Input: part model. Units: mm. Frame: model coordinates. A direction names the side the tool comes from. Coordinates: 2 decimals unless noted, no trailing zeros. Loops run counter-clockwise (first coordinate to the right, second up) from the corner with the lowest first, then second, coordinate; pieces in that order, holes last. Notation, with made-up numbers: M 84.25,43.5 L 123.25,43.5 A34 cw 123.25,73.5 Z; hole C 15.25,76.25 d5. An arc over 180 degrees is marked long. Use a Markdown table: item, result. Add a question column.
1. Pin query (flat end, axial travel): pin 1 (4 mm diameter, centred on x = 86.5, y = 23.5, fed in from +Z); pin 2 (4 mm diameter, centred on x = 32.5, y = 26.5, fed in from -Z); pin 3 (2 mm diameter, centred on x = 104, y = 16.5, fed in from +Z). Return the tip coordinate at first contact, or that it passes through.
2. Line query: L1, parallel to Y at x = 115, z = -24; L2, parallel to Z at x = 47.5, y = 40; L3, parallel to X at y = 10, z = 34.5. Output: solid intervals per line, ascending. Write a range as [from, to].
3. Section C-C on x = 112. Output: boundary loops of the cut face in (y, z), then the cut area to 3 significant figures.
4. Section A-A on y = 7. Output: boundary loops of the cut face in (x, z), then the cut area to 3 significant figures.
5. Set-up query: faces 1 (the flat face through (112, 22, 23)), 2 (the flat face through (105, 0, -23)). Return all of +Z, -Z, +X, -X, +Y, -Y with unobstructed straight access to the full face (end or side cutting, diameter ignored); none if empty.
6. Section D-D on y = 22. Output: boundary loops of the cut face in (x, z).
7. Section B-B on z = 46.5. Output: boundary loops of the cut face in (x, y).
```python
from build123d import *

# Parameters (mm, degrees)
SURFACESAB_DEPTH        = 150
SURFACESCD_DEPTH        = 80
SURFACESCD_DEPTH_BACK   = 70
CUT_EXTRUDE3_DEPTH      = 42.711375741
SURFACEE_DEPTH          = 130
CUT_EXTRUDE9_DEPTH      = 81
CUT_EXTRUDE9_DEPTH_BACK = 71
CUT_EXTRUDE10_DEPTH     = 150


with BuildPart() as part:
    # Sketch2 → SurfacesAB (new body)
    with BuildSketch(Plane(origin=(0, 0, 0), x_dir=(0, 0, -1), z_dir=(1, 0, 0))):
        Polygon((0, 0), (35, 41.711375741), (70, 0), align=None)
    extrude(amount=SURFACESAB_DEPTH)

    # Sketch3 → SurfacesCD (add, two sides)
    with BuildSketch(Plane.XY) as surfacescd_sk:
        Polygon((150, 0), (120, 30), (90, 0), align=None)
    extrude(amount=SURFACESCD_DEPTH)
    extrude(surfacescd_sk.sketch, amount=-SURFACESCD_DEPTH_BACK)

    # Sketch6 → Cut-Extrude3 (cut, through all)
    with BuildSketch(Plane(origin=(0, 0, 0), x_dir=(1, 0, 0), z_dir=(0, 1, 0))):
        Polygon((0, 70), (150, -80), (0, -80), align=None)
    extrude(amount=CUT_EXTRUDE3_DEPTH, mode=Mode.SUBTRACT)

    # Sketch13 → SurfaceE (add)
    with BuildSketch(Plane(origin=(150, 0, 80), x_dir=(-0.707106781, 0, 0.707106781), z_dir=(-0.707106781, 0, -0.707106781))):
        Polygon((0, 0), (-14.142135624, 0), (-79.799705645, 50.488741568), (-80.104771591, 61.598214949), align=None)
    extrude(amount=SURFACEE_DEPTH)

    # Sketch10 → Cut-Extrude9 (cut, two sides)
    with BuildSketch(Plane.XY) as cut_extrude9_sk:
        Polygon((150, 0), (83.43213667, 66.56786333), (150, 66.56786333), (213.23579194, 66.56786333), (213.23579194, 0), align=None)
    extrude(amount=CUT_EXTRUDE9_DEPTH, mode=Mode.SUBTRACT)
    extrude(cut_extrude9_sk.sketch, amount=-CUT_EXTRUDE9_DEPTH_BACK, mode=Mode.SUBTRACT)

    # Sketch4 → Cut-Extrude10 (cut)
    with BuildSketch(Plane(origin=(150, 0, 0), x_dir=(0, 0, -1), z_dir=(1, 0, 0))):
        Polygon((70, 0), (18.686100405, 61.153524192), (70, 61.153524192), align=None)
    extrude(amount=-CUT_EXTRUDE10_DEPTH, mode=Mode.SUBTRACT)


solid = part.part
```
Answers below:
| question | item | result |
|---|---|---|
| 1 | pin 1 | stops at z = -18.04 |
| 1 | pin 2 | stops at z = -49.44 |
| 1 | pin 3 | stops at z = 5.75 |
| 2 | L1 | y = [0, 35] |
| 2 | L2 | z = [-36.44, -33.56] |
| 2 | L3 | x = [104.5, 140] |
| 3 | outline | M 0,-70 L 38,-38.11 L 38,-27.89 L 22,1.54 L 22,42 L 0,42 Z |
| 3 | area | 2,770 mm² |
| 4 | outline | M 5.87,-64.13 L 143,-64.13 L 143,73 L 97,27 L 97,14.13 L 77,-5.87 L 64.13,-5.87 Z |
| 4 | area | 9,060 mm² |
| 5 | face 1 | +Z, -X, +Y |
| 5 | face 2 | +Z, -Z, +X, -X, -Y |
| 6 | outline | M 18.46,-51.54 L 128,-51.54 L 128,58 L 112,42 L 112,1.54 L 92,-18.46 L 51.54,-18.46 Z |
| 7 | outline | M 116.5,0 L 150,0 L 120,30 L 116.5,26.5 Z |
